```python
from build123d import *

# Parameters (mm, degrees)
F4_R = 1.190625
F5_R = 1.190625


with BuildPart() as f3:
    # F2 (on Front) → F3 (revolve)
    with BuildSketch(Plane.XZ):
        Polygon((-1.5875, -3.175), (-1.5875, 3.175), (-5.5626, 3.175), (-5.5626, 1.5875), (-3.96875, 1.5875), (-3.96875, -1.5875), (-5.5626, -1.5875), (-5.5626, -3.175), align=None)
    revolve(axis=Axis((0, 0, 0.0240590106), (0, 0, -1)))

    # F4
    f4_edges = [f3.edges().sort_by_distance(p)[0] for p in [
        (5.5626, 0, 3.175),
    ]]
    fillet(f4_edges, radius=F4_R)

    # F5
    f5_edges = [f3.edges().sort_by_distance(p)[0] for p in [
        (5.5626, 0, -3.175),
    ]]
    fillet(f5_edges, radius=F5_R)


solid = f3.part
```
Can you work these out from the model? Positions are in its coordinate system, mm. A direction names the side the tool comes from. Round coordinates to 2 decimals unless told otherwise and drop trailing zeros. Order: outer loops, then holes, each group sorted by start corner. A loop starts at its lowest first (then second) coordinate and runs counter-clockwise, first axis right, second up.
(1) If we section it at C-C (z = -1): Please give me the cut outline in (x, y) (1 decimal).
Results are:
outline: circle Ø7.9 at (0, 0); hole circle Ø3.2 at (0, 0)
(2) If I drill on L1, parallel to Z at x = -3.5, y = -2.5 (1 decimal); L2, parallel to Y at x = 0, z = -1; L3, parallel to Y at x = 0, z = 1.75, over which ranges is the centre line in solid material (lowest first)?
Results are:
L1: z = -3.2 to -1.6, 1.6 to 3.2
L2: y = -3.97 to -1.59, 1.59 to 3.97
L3: y = -5.56 to -1.59, 1.59 to 5.56
(3) On a 3-axis mill with a long thin cutter (end or side, diameter ignored), from which of +Z, -Z, +X, -X, +Y, -Y can I reach the whole of each face in a straight line? I mean faces 1 (the face through (0, -2, 3.175)), 2 (the face through (-4, 1, -1.588)). Say none if no direction works.
Results are:
face 1: +Z, +X, -X, +Y, -Y
face 2: none
(4) We'd pull the mould along Z, two halves only. Please class faces 3 (the face through (0, -2, -3.175)), 4 (the face through (4, 1, 1.588)), 5 (the face through (0.86, -3.874, -0.022)), 6 (the face through (-5.306, 1.671, 1.783)): +Z half, -Z half, draft (parallel to the pull), parting line (faces both ways), or undercut.
Results are:
face 3: -Z half
face 4: undercut
face 5: undercut
face 6: draft
